from build123d import *

# Parameters (mm, degrees)
CROQUIS1_R              = 11
CROQUIS1_R_2            = 2
CROQUIS1_W              = 30
CROQUIS1_H              = 3
SALIENTE_EXTRUIR1_DEPTH = 3
CROQUIS2_R              = 13
CROQUIS2_R_2            = 11
SALIENTE_EXTRUIR2_DEPTH = 4
CROQUIS3_R              = 13
CROQUIS3_R_2            = 9
SALIENTE_EXTRUIR3_DEPTH = 2
CHAFL_N1_SIZE           = 2
CHAFL_N2_SIZE           = 10
CROQUIS4_W              = 10
CROQUIS4_H              = 20
CROQUIS4_R              = 2.5
SALIENTE_EXTRUIR4_DEPTH = 1.5


with BuildPart() as part:
    # Croquis1 → Saliente-Extruir1 (new body)
    with BuildSketch(Plane(origin=(0, 0, 0), x_dir=(1, 0, 0), z_dir=(0, 1, 0))):
        Polygon((-67.5, -20), (67.5, -20), (67.5, 20), (-67.5, 20), (-67.5, 10), (-57.5, 10), (-57.5, -10), (-67.5, -10), align=None)
        with Locations(Location((48.5, 0, 0), (0, 0, 270))):
            Circle(CROQUIS1_R, mode=Mode.SUBTRACT)
        with Locations(Location((-52.5, 0, 0), (0, 0, 270))):
            Circle(CROQUIS1_R_2, mode=Mode.SUBTRACT)
        with Locations(Location((23.5, 0, 0), (0, 0, 270))):
            Circle(CROQUIS1_R_2, mode=Mode.SUBTRACT)
        with Locations(Location((8.5, 0, 0), (0, 0, 270))):
            Circle(CROQUIS1_R_2, mode=Mode.SUBTRACT)
        with Locations((-27.5, 11)):
            Rectangle(CROQUIS1_W, CROQUIS1_H, mode=Mode.SUBTRACT)
        with Locations((-27.5, -11)):
            Rectangle(CROQUIS1_W, CROQUIS1_H, mode=Mode.SUBTRACT)
    extrude(amount=SALIENTE_EXTRUIR1_DEPTH)

    # Croquis2 → Saliente-Extruir2 (add)
    with BuildSketch(Plane(origin=(0, 3, 0), x_dir=(1, 0, 0), z_dir=(0, 1, 0))):
        with Locations(Location((48.5, 0, 0), (0, 0, 90))):
            Circle(CROQUIS2_R)
        with Locations(Location((48.5, 0, 0), (0, 0, 270))):
            Circle(CROQUIS2_R_2, mode=Mode.SUBTRACT)
    extrude(amount=SALIENTE_EXTRUIR2_DEPTH)

    # Croquis3 → Saliente-Extruir3 (add)
    with BuildSketch(Plane(origin=(0, 7, 0), x_dir=(1, 0, 0), z_dir=(0, 1, 0))):
        with Locations(Location((48.5, 0, 0), (0, 0, 90))):
            Circle(CROQUIS3_R)
        with Locations(Location((48.5, 0, 0), (0, 0, 270))):
            Circle(CROQUIS3_R_2, mode=Mode.SUBTRACT)
    extrude(amount=SALIENTE_EXTRUIR3_DEPTH)

    # Chaflán1
    chafl_n1_edges = [part.edges().sort_by_distance(p)[0] for p in [
        (48.5, 9, 13),
    ]]
    chamfer(chafl_n1_edges, length=CHAFL_N1_SIZE)

    # Chaflán2
    chafl_n2_edges = [part.edges().sort_by_distance(p)[0] for p in [
        (67.5, 1.5, 20),
        (67.5, 1.5, -20),
    ]]
    chamfer(chafl_n2_edges, length=CHAFL_N2_SIZE)

    # Croquis4 → Saliente-Extruir4 (add)
    with BuildSketch(Plane(origin=(0, 3, 0), x_dir=(1, 0, 0), z_dir=(0, 1, 0))):
        with Locations((-62.5, 0)):
            Rectangle(CROQUIS4_W, CROQUIS4_H)
        with Locations(Location((-62.5, 0, 0), (0, 0, 270))):
            Circle(CROQUIS4_R, mode=Mode.SUBTRACT)
    extrude(amount=-SALIENTE_EXTRUIR4_DEPTH)


solid = part.part
The model under review builds one solid part; all positions refer to its coordinate system, in mm. A direction names the side the tool comes from. Round coordinates to 2 decimals unless told otherwise and drop trailing zeros. Order: outer loops, then holes, each group sorted by start corner. A loop starts at its lowest first (then second) coordinate and runs counter-clockwise, first axis right, second up. Notation, with made-up numbers: (-6.75, 50.25) - (23.25, 50.25) arc R23 ccw to (23.25, 77.25) - close; hole circle Ø1 at (64, -34.75). An arc over 180 degrees is marked (long way). Use one line per item in the form item = value.
Q1. Add section A-A on x = 8.5. Give the boundary of the cut face in (y, z).
Response values:
outline = (0, -20) - (3, -20) - (3, -2) - (0, -2) - close; (0, 2) - (3, 2) - (3, 20) - (0, 20) - close
Q2. Mouldability with a two-part tool opening along Z and no side actions: class faces 1 (the flat face through (57, 9, 4)), 2 (the flat face through (-12.5, 1, 11)), 3 (the flat face through (-4, 1, -20)) as pulls with the +Z half, pulls with the -Z half, needs draft (parallel to the pull), parting line crosses it, or undercut.
Response values:
face_1 = needs draft
face_2 = undercut
face_3 = pulls with the -Z half
Q3. Add section B-B on x = -14.5. Give the boundary of the cut face in (y, z), then the cut area to 3 significant figures.
Response values:
outline = (0, -20) - (3, -20) - (3, -12.5) - (0, -12.5) - close; (0, -9.5) - (3, -9.5) - (3, 9.5) - (0, 9.5) - close; (0, 12.5) - (3, 12.5) - (3, 20) - (0, 20) - close
area = 102 mm^2
Q4. Add section D-D on z = 0. Give the number of separate pieces and of enclosed holes in the cut face, then the cut area to 4 significant figures.
Response values:
separate_pieces = 6
enclosed_holes = 0
area = 308.5 mm^2
Q5. Clearance check with flat-ended pins moving along their axes: P1, Ø1, axis at x = 14, z = -9.5, coming from the +Y side; P2, Ø5, axis at x = -61.5, z = 4.5, coming from the -Y side; P3, Ø0.9, axis at y = 1, z = 11.5, coming from the +X side. State where each tip first meets the part, or that it passes through.
Response values:
P1 = 3
P2 = 1.5
P3 = 66.45
Q6. Tool access review of faces 4 (the cylindrical face through (59.406, 3.451, -1.432)), 5 (the flat face through (-63.7, 1.5, -2.4)), 6 (the flat face through (-42.5, 1, -11)), 7 (the cylindrical face through (35.61, 4.97, 1.69)): name each direction out of +Z, -Z, +X, -X, +Y, -Y from which nothing blocks a thin tool from reaching the whole face with its end or side.
Response values:
face_4 = -Y
face_5 = -X, -Y
face_6 = +Y, -Y
face_7 = +Y
Q7. To check wall thickness, follow line 1 (X direction, y = 0.95, z = 0); line 2 (X direction, y = 2, z = 0); line 3 (Y direction, x = -16.5, z = 5). State the ranges of each line that lie inside material, in increasing order.
Response values:
line_1 = -57.5 to -54.5, -50.5 to 6.5, 10.5 to 21.5, 25.5 to 37.5, 59.5 to 67.5
line_2 = -67.5 to -65, -60 to -54.5, -50.5 to 6.5, 10.5 to 21.5, 25.5 to 37.5, 59.5 to 67.5
line_3 = 0 to 3
Q8. Add section C-C on y = 5. Give the boundary of the cut face in (x, z), then the cut area to 3 significant figures.
Response values:
outline = circle Ø26 at (48.5, 0); hole circle Ø22 at (48.5, 0)
area = 151 mm^2
